Model file for the job. Use its own axes, mm. Coordinates: 2 decimals unless noted, no trailing zeros. Order: outer loops, then holes, each group sorted by start corner. A loop starts at its lowest first (then second) coordinate and runs counter-clockwise, first axis right, second up.
from build123d import *

# Parameters (mm, degrees)
SKETCH2_W           = 300
SKETCH2_H           = 30
BOSS_EXTRUDE1_DEPTH = 5
SKETCH3_R           = 4
SKETCH3_R_2         = 10
CUT_EXTRUDE1_DEPTH  = 5
SKETCH5_R           = 2
CUT_EXTRUDE2_DEPTH  = 5


with BuildPart() as part:
    # Sketch2 → Boss-Extrude1 (new body)
    with BuildSketch(Plane(origin=(0, 0, 0), x_dir=(1, 0, 0), z_dir=(0, 1, 0))):
        Rectangle(SKETCH2_W, SKETCH2_H)
    extrude(amount=BOSS_EXTRUDE1_DEPTH)

    # Sketch3 → Cut-Extrude1 (cut)
    with BuildSketch(Plane(origin=(0, 5, 0), x_dir=(1, 0, 0), z_dir=(0, 1, 0))):
        with Locations((-135, 0)):
            Circle(SKETCH3_R)
        Circle(SKETCH3_R_2)
        with Locations((135, 0)):
            Circle(SKETCH3_R)
    extrude(amount=-CUT_EXTRUDE1_DEPTH, mode=Mode.SUBTRACT)

    # Sketch5 → Cut-Extrude2 (cut)
    with BuildSketch(Plane(origin=(0, 5, 0), x_dir=(1, 0, 0), z_dir=(0, 1, 0))):
        with Locations((100, 0)):
            Circle(SKETCH5_R)
        with Locations((-100, 0)):
            Circle(SKETCH5_R)
    extrude(amount=-CUT_EXTRUDE2_DEPTH, mode=Mode.SUBTRACT)


solid = part.part
Q1. Cut at C-C, the plane z = 7.5. List the corners of the cut face in (x, y).
Established:
outline: (-150, 0) - (-6.61, 0) - (-6.61, 5) - (-150, 5) - close; (6.61, 0) - (150, 0) - (150, 5) - (6.61, 5) - close
Q2. Cut at B-B, the plane y = 3.1. List the corners of the cut face in (x, z).
Established:
outline: (-150, -15) - (150, -15) - (150, 15) - (-150, 15) - close; hole circle Ø8 at (-135, 0); hole circle Ø4 at (-100, 0); hole circle Ø20 at (0, 0); hole circle Ø4 at (100, 0); hole circle Ø8 at (135, 0)
Q3. Probe line 1 (X direction, y = 2.75, z = 0); line 2 (Z direction, x = 134.5, y = 0.3); line 3 (Z direction, x = -100, y = 3.2). List the from-to ranges inside material, lowest first.
Established:
line 1: x = -150 to -139, -131 to -102, -98 to -10, 10 to 98, 102 to 131, 139 to 150
line 2: z = -15 to -3.97, 3.97 to 15
line 3: z = -15 to -2, 2 to 15
Q4. Drop flat-ended pins along their axis: P1, Ø3.5, axis at x = 100, z = 0, coming from the -Y side; P2, Ø12, axis at x = -104, z = -8.5, coming from the -Y side. Give the stop position or say it passes through.
Established:
P1: passes through
P2: stops at y = 0
Q5. Cut at A-A, the plane x = 0. List the corners of the cut face in (y, z).
Established:
outline: (0, -15) - (5, -15) - (5, -10) - (0, -10) - close; (0, 10) - (5, 10) - (5, 15) - (0, 15) - close
Q6. Mould opens along X. For faces 1 (the face through (150, 2, 0)), 2 (the face through (-2, 2, -15)), 3 (the face through (-131.185, 2.535, -1.201)) say: pulls with the +X half, pulls with the -X half, needs draft (parallel to the pull), parting line crosses it, or undercut.
Established:
face 1: pulls with the +X half
face 2: needs draft
face 3: undercut
